The figure shows three views and two pictorial views of one solid part (mm, origin at its lowest corner). Answer the questions. A direction names the side the tool comes from. Round coordinates to 2 decimals unless told otherwise and drop trailing zeros. Write each loop counter-clockwise with the first axis right and the second up, starting at its lowest first coordinate (ties: lowest second). Pieces come first, ordered by that corner, then holes. Notation, with made-up numbers: (85.25, -28.5) -> (121.25, -28.5) arc R16 ccw to (121.25, -17.5) -> close; hole circle Ø4 at (52.5, -8.75). An arc over 180 degrees is marked (long way). One line per item, written item: value.
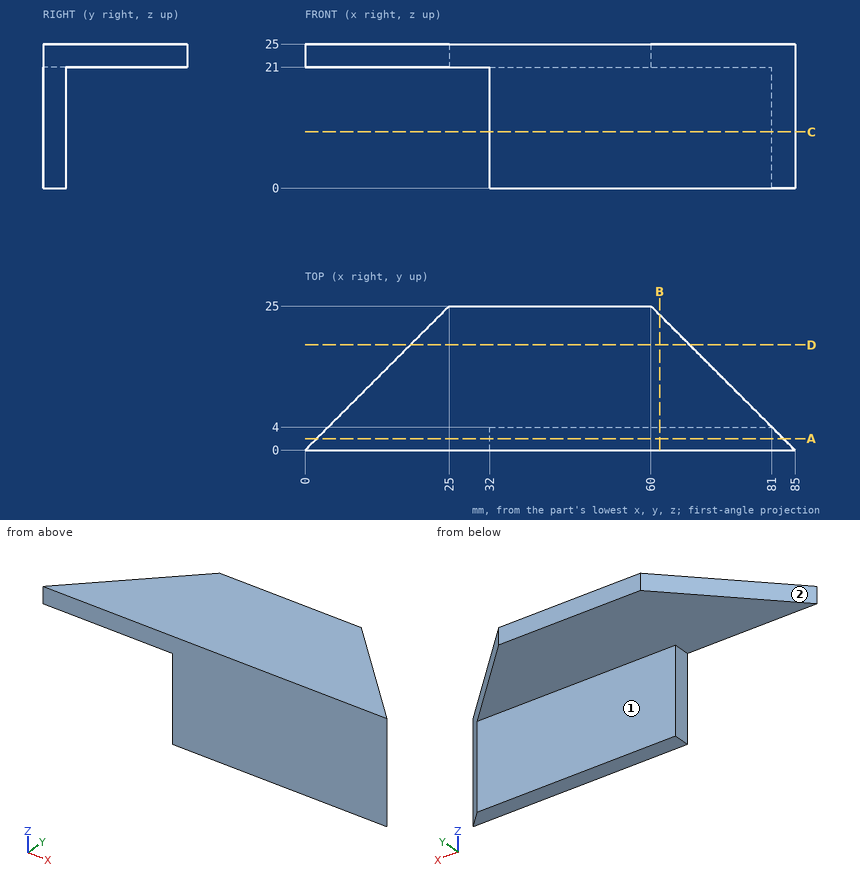
(1) A tool of negligible diameter and unlimited length cuts with its end or side. For the marked faces 1 and 2, from which of +Z, -Z, +X, -X, +Y, -Y can it reach the whole face along a straight path? Write none if from no direction.
Reported:
face 1: -Z, +X, -X, +Y
face 2: +Z, -Z, -X, +Y
(2) Flat-ended cylindrical pins translate along their axes: pin 1 Ø1.5 at (x, y) = (60, 5) entering from -Z; pin 2 Ø12 at (y, z) = (13.5, 3) entering from -X; pin 3 Ø1.2 at (y, z) = (1.5, 8) entering from -X; pin 4 Ø12 at (x, z) = (48.5, 17.5) entering from +Y. Find the tip coordinate at first contact, or state that the pin passes through.
Reported:
pin 1: stops at z = 21
pin 2: passes through
pin 3: stops at x = 32
pin 4: stops at y = 25
(3) Find section A-A on y = 2. Give the vertices of the cut face in (x, z).
Reported:
outline: (2, 21) -> (32, 21) -> (32, 0) -> (83, 0) -> (83, 25) -> (2, 25) -> close
(4) Find section C-C on z = 9.75. Give the vertices of the cut face in (x, y), plus the area to 3 significant figures.
Reported:
outline: (32, 0) -> (85, 0) -> (81, 4) -> (32, 4) -> close
area: 204 mm2
(5) Consider probe 1 along Z at (x, y) = (67, 6.5); probe 2 along Y at (x, z) = (51.5, 20.75); probe 3 along X at (y, z) = (1.5, 3.5). Determine where each line is inside the solid, lowest interval first.
Reported:
probe 1: z = 21 to 25
probe 2: y = 0 to 4
probe 3: x = 32 to 83.5
(6) Find section D-D on y = 18.25. Give the vertices of the cut face in (x, z).
Reported:
outline: (18.25, 21) -> (66.75, 21) -> (66.75, 25) -> (18.25, 25) -> close
(7) Find section B-B on x = 61.5. Give the vertices of the cut face in (y, z), plus the area to 3 significant figures.
Reported:
outline: (0, 0) -> (4, 0) -> (4, 21) -> (23.5, 21) -> (23.5, 25) -> (0, 25) -> close
area: 178 mm2
